from build123d import *

# Parameters (mm, degrees)
EXTRUDE_1_DEPTH     = 180
SKETCH_4_W          = 115.68849301
SKETCH_4_H          = 90
CUT_EXTRUDE_1_DEPTH = 200


with BuildPart() as part:
    # 草图1 → 凸台-拉伸1 (new body)
    with BuildSketch(Plane(origin=(0, 0, 0), x_dir=(1, 0, 0), z_dir=(0, 1, 0))):
        Polygon((-18.406325618, 0), (61.985157699, 0), (81.593674382, 17.5), (61.985157699, 35), (26.593674382, 35), (26.593674382, 59.919439784), (4.093674382, 80), (-18.406325618, 59.919439784), align=None)
    extrude(amount=EXTRUDE_1_DEPTH)

    # 草图4 → 切除-拉伸1 (cut)
    with BuildSketch(Plane(origin=(26.593674382, 0, 0), x_dir=(0, 0, -1), z_dir=(1, 0, 0))):
        with Locations((92.844246505, 45)):
            Rectangle(SKETCH_4_W, SKETCH_4_H)
    extrude(amount=-CUT_EXTRUDE_1_DEPTH, mode=Mode.SUBTRACT)


solid = part.part
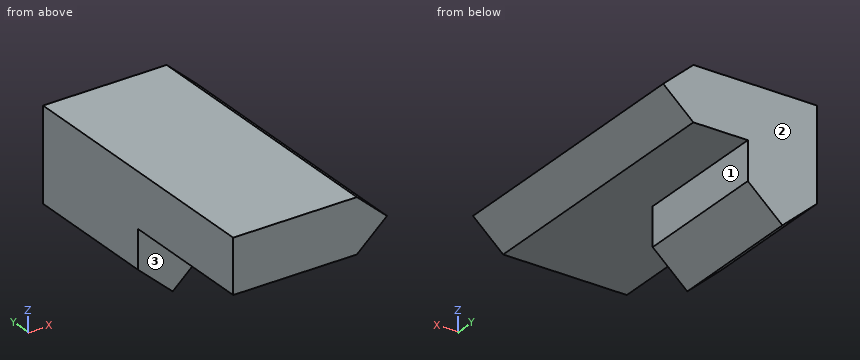
Could you check a few things on this model? Use its own coordinates, in mm. Face numbers are marked on the shaded views. A direction names the side the tool comes from. Coordinates: 2 decimals unless noted, no trailing zeros. Order: outer loops, then holes, each group sorted by start corner. A loop starts at its lowest first (then second) coordinate and runs counter-clockwise, first axis right, second up. Notation, with made-up numbers: (-25.75, 9) - (-3.75, 9) arc R9 ccw to (-3.75, 13) - close; hole circle Ø11 at (-14.5, 85). An arc over 180 degrees is marked (long way). Answer in a Markdown table with one row per item. Add a question column.
(1) If we section it at D-D, the plane y = 32: Please give me the cut outline in (x, z).
(2) If we section it at C-C, the plane x = -0.5: Please give me the cut outline in (y, z).
(3) Will these pins go through, and if not, where does the flat tip stop? pin 1 (3 mm diameter, centred on x = 22.5, z = -65.5, fed in from -Y); pin 2 (4 mm diameter, centred on x = 47, y = 71, fed in from -Z); pin 3 (4 mm diameter, centred on x = 31.5, y = 18.5, fed in from +Z); pin 4 (4 mm diameter, centred on x = 66, y = 66, fed in from +Z).
(4) On a 3-axis mill with a long thin cutter (end or side, diameter ignored), from which of +Z, -Z, +X, -X, +Y, -Y can I reach the whole of each face in a straight line? I mean the marked faces 1, 2 and 3. Say none if no direction works.
(5) If we section it at A-A, the plane y = 105: Please give me the cut outline in (x, z).
(6) I need wall thicknesses on L1, parallel to Z at x = 41, y = 45; L2, parallel to Y at x = 12, z = -53.5; L3, parallel to X at y = 160, z = -48. Which ranges of each line are inside material? Lowest first, please.
(7) If we section it at B-B, the plane z = -56: Please give me the cut outline in (x, y).
Results are:
| question | item | result |
|---|---|---|
| 1 | outline | (-18.41, -35) - (61.99, -35) - (81.59, -17.5) - (61.99, 0) - (-18.41, 0) - close |
| 2 | outline | (0, -35) - (90, -35) - (90, -75.9) - (180, -75.9) - (180, 0) - (0, 0) - close |
| 3 | pin 1 | stops at y = 90 |
| 3 | pin 2 | stops at z = -35 |
| 3 | pin 3 | stops at z = 0 |
| 3 | pin 4 | stops at z = -1.8 |
| 4 | face 1 | -Z, +X, +Y, -Y |
| 4 | face 2 | +Z, -Z, +X, -X, +Y |
| 4 | face 3 | -Z, +X, -X, -Y |
| 5 | outline | (-18.41, -59.92) - (4.09, -80) - (26.59, -59.92) - (26.59, -35) - (61.99, -35) - (81.59, -17.5) - (61.99, 0) - (-18.41, 0) - close |
| 6 | L1 | z = -35 to 0 |
| 6 | L2 | y = 90 to 180 |
| 6 | L3 | x = -18.41 to 26.59 |
| 7 | outline | (-18.41, 90) - (26.59, 90) - (26.59, 180) - (-18.41, 180) - close |
